from build123d import *

# Parameters (mm, degrees)
SKETCH1_W               = 380
SKETCH1_H               = 195
BOSS_EXTRUDE1_DEPTH     = 21
FILLET1_R               = 99
SKETCH2_W               = 101
SKETCH2_H               = 20
CUT_EXTRUDE1_DEPTH      = 13
FILLET2_R               = 4
CUT_EXTRUDE2_DEPTH      = 110
CUT_EXTRUDE2_DEPTH_BACK = 10
SKETCH3_R               = 3
SKETCH4_W               = 99
SKETCH4_H               = 21
BOSS_EXTRUDE2_DEPTH     = 49
FILLET3_R               = 24


with BuildPart() as part:
    # Sketch1 → Boss-Extrude1 (new body)
    with BuildSketch(Plane(origin=(0, 0, 0), x_dir=(1, 0, 0), z_dir=(0, 1, 0))):
        Rectangle(SKETCH1_W, SKETCH1_H)
    extrude(amount=BOSS_EXTRUDE1_DEPTH)

    # Fillet1
    # the kernel refuses this fillet: 99 mm, written as the material it takes off along each edge
    with BuildSketch(Plane(origin=(-190, -247.5, 97.5), x_dir=(0, 0, -1), z_dir=(0, 1, 0)), Plane(origin=(-190, -247.5, -97.5), x_dir=(1, 0, 0), z_dir=(0, 1, 0)), Plane(origin=(190, -247.5, 97.5), x_dir=(-1, 0, 0), z_dir=(0, 1, 0))) as fillet1_piece_1:
        with BuildLine():
            CenterArc((FILLET1_R, -FILLET1_R), FILLET1_R, 90, 90)
            Line((0, -FILLET1_R), (0, 0))
            Line((0, 0), (FILLET1_R, 0))
        make_face()
    extrude(amount=516, mode=Mode.SUBTRACT)
    with BuildSketch(Plane(origin=(190, -247.5, -97.5), x_dir=(-1, 0, 0), z_dir=(0, 1, 0))) as fillet1_piece_2:
        with BuildLine():
            CenterArc((FILLET1_R, FILLET1_R), FILLET1_R, 180, 90)
            Line((0, FILLET1_R), (0, 0))
            Line((0, 0), (FILLET1_R, 0))
        make_face()
    extrude(amount=516, mode=Mode.SUBTRACT)

    # Sketch2 → Cut-Extrude1 (cut)
    with BuildSketch(Plane.XZ):
        with Locations((0, 97.5)):
            Rectangle(SKETCH2_W, SKETCH2_H)
    extrude(amount=-CUT_EXTRUDE1_DEPTH, mode=Mode.SUBTRACT)

    # Fillet2
    fillet2_edges = [part.edges().sort_by_distance(p)[0] for p in [
        (0, 13, 87.5),
    ]]
    fillet(fillet2_edges, radius=FILLET2_R)

    # Sketch3 → Cut-Extrude2 (cut, two sides: drawn at the far end of the back side and taken through both)
    with BuildSketch(Plane(origin=(-50.5, 0, 0), x_dir=(0, 0, -1), z_dir=(1, 0, 0)).offset(-CUT_EXTRUDE2_DEPTH_BACK)):
        with Locations((-92.5, 8)):
            Circle(SKETCH3_R)
    extrude(amount=CUT_EXTRUDE2_DEPTH + CUT_EXTRUDE2_DEPTH_BACK, mode=Mode.SUBTRACT)

    # Sketch4 → Boss-Extrude2 (add)
    with BuildSketch(Plane(origin=(0, 0, -97.5), x_dir=(-1, 0, 0), z_dir=(0, 0, -1))):
        with Locations((0, 10.5)):
            Rectangle(SKETCH4_W, SKETCH4_H)
    extrude(amount=BOSS_EXTRUDE2_DEPTH)

    # Fillet3
    fillet3_edges = [part.edges().sort_by_distance(p)[0] for p in [
        (49.5, 10.5, -146.5),
        (-49.5, 10.5, -146.5),
    ]]
    fillet(fillet3_edges, radius=FILLET3_R)


solid = part.part
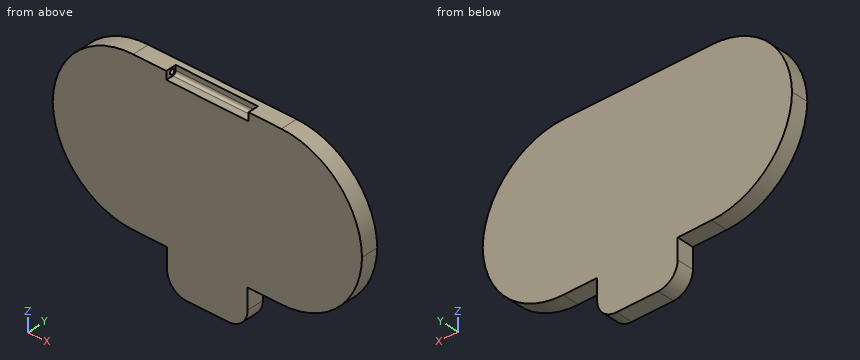
Geometry check sheet. Reference: the model listing, model coordinates, mm. Give positions to 0.01 mm unless a question says otherwise; leave off trailing zeros. Write each loop counter-clockwise with the first axis right and the second up, starting at its lowest first coordinate (ties: lowest second). Pieces come first, ordered by that corner, then holes. Notation, with made-up numbers: (-17.5, 82.5) - (15.5, 82.5) arc R32 ccw to (15.5, 120.5) - close; hole circle Ø4 at (77, 49.5). An arc over 180 degrees is marked (long way). Put each result on its own line as item: value.
1. Sectioned sample at B-B, the plane z = -55. Enter the section's corners in (x, y).
Ans:
outline: (-172.29, 0) - (172.29, 0) - (172.29, 21) - (-172.29, 21) - close
2. Sectioned sample at A-A, the plane x = -12. Enter the section's corners in (y, z).
Ans:
outline: (0, -146.5) - (21, -146.5) - (21, 97.5) - (13, 97.5) - (13, 91.5) arc R4 cw to (9, 87.5) - (0, 87.5) - close
3. Go/stop test with flat-tipped pins: pin 1 (11 mm diameter, centred on y = 4, z = 93.5, fed in from -X); pin 2 (2 mm diameter, centred on y = 14.5, z = -108.5, fed in from +X); pin 3 (6.5 mm diameter, centred on y = 15.5, z = -115.5, fed in from -X); pin 4 (3 mm diameter, centred on x = -11, z = -5.5, fed in from -Y). Record where each tip stops, or that it passes through.
Ans:
pin 1: stops at x = -133.32
pin 2: stops at x = 49.5
pin 3: stops at x = -49.5
pin 4: stops at y = 0
4. Thickness scan on line 1 (Y direction, x = 55.5, z = 92.5); line 2 (Z direction, x = 57, y = 8); line 3 (Z direction, x = 79.5, y = 14.25). Record the ranges inside material, lowest first.
Ans:
line 1: y = 0 to 5, 11 to 21
line 2: z = -97.5 to 89.5, 95.5 to 97.5
line 3: z = -97.5 to 97.5
5. Sectioned sample at C-C, the plane x = -97.5. Enter the section's corners in (y, z), plus the area to 3 significant figures.
Ans:
outline: (0, -97.29) - (21, -97.29) - (21, 97.29) - (0, 97.29) - close
area: 4,090 mm²
